Geometry: final body of the model. Coordinates: model frame, mm. A direction names the side the tool comes from. Give positions to 0.01 mm unless a question says otherwise; leave off trailing zeros. Order: outer loops, then holes, each group sorted by start corner. A loop starts at its lowest first (then second) coordinate and runs counter-clockwise, first axis right, second up. Notation, with made-up numbers: (83.25, 17) - (134.25, 17) arc R34 ccw to (134.25, 50) - close; hole circle Ø7 at (30.5, 56). An arc over 180 degrees is marked (long way). One line per item, written item: value.
```python
from build123d import *

# Parameters (mm, degrees)
F1_DEPTH = 12.7
F2_DEPTH = 25.4
F3_DEPTH = 50.8


with BuildPart() as f1:
    # F0 (on Front) → F1 (new body)
    with BuildSketch(Plane.XZ):
        Polygon((23.827744, -32.507298), (27.511551, -30.380452), (11.636551, -2.884145), (7.952744, -5.010992), (-7.922256, -32.507298), align=None)
        Polygon((27.511551, -30.380452), (32.624925, -29.077077), (18.205816, -4.102446), (11.636551, -2.884145), align=None)
    extrude(amount=-F1_DEPTH)

    # F0 (on Front) → F2 (join)
    with BuildSketch(Plane.XZ):
        with BuildLine():
            Line((32.624925, -29.077077), (36.2911, -22.727077))
            Line((36.2911, -22.727077), (23.705077, -0.927446))
            ThreePointArc((23.705077, -0.927446), (24.022261, -1.693196), (24.130446, -2.514946))
            ThreePointArc((24.130446, -2.514946), (21.777197, -5.581761), (18.205816, -4.102446))
            Line((18.205816, -4.102446), (32.624925, -29.077077))
        make_face()
    extrude(amount=-F2_DEPTH)

    # F0 (on Front) → F3 (join)
    with BuildSketch(Plane.XZ):
        with BuildLine():
            ThreePointArc((24.130446, -2.514946), (24.022261, -1.693196), (23.705077, -0.927446))
            ThreePointArc((23.705077, -0.927446), (19.367946, 0.234685), (18.205816, -4.102446))
            ThreePointArc((18.205816, -4.102446), (21.777197, -5.581761), (24.130446, -2.514946))
        make_face()
    extrude(amount=-F3_DEPTH)


solid = f1.part
```
1) Section D-D, the plane y = 23. Return loops of the section in (x, z) (3 decimals), then the cut area to 3 significant figures.
Answers below:
outline: (18.206, -4.102) - (32.625, -29.077) - (36.291, -22.727) - (23.705, -0.927) arc R3.175 ccw to start
area: 187 mm^2
2) Section C-C, the plane z = -25. Return loops of the section in (x, y), then the cut area to 3 significant figures.
Answers below:
outline: (-3.59, 0) - (34.98, 0) - (34.98, 25.4) - (30.27, 25.4) - (30.27, 12.7) - (-3.59, 12.7) - close
area: 550 mm^2
3) Section B-B, the plane x = 22. Return loops of the section in (y, z), then the cut area to 3 significant figures.
Answers below:
outline: (0, -32.51) - (12.7, -32.51) - (12.7, -10.67) - (25.4, -10.67) - (25.4, -5.51) - (50.8, -5.51) - (50.8, 0.48) - (0, 0.48) - close
area: 713 mm^2
4) First-contact query: pin 1 (1.5 mm diameter, centred on x = 2, z = -25.5, fed in from +Y); pin 2 (9 mm diameter, centred on x = 22, z = -18, fed in from +Y); pin 3 (1.5 mm diameter, centred on y = 40, z = -6.5, fed in from -X); pin 4 (10 mm diameter, centred on y = 19, z = -7.5, fed in from -X). Flat tips, straight axial feed; report the tip coordinate or a pass-through.
Answers below:
pin 1: y = 12.7
pin 2: y = 25.4
pin 3: through
pin 4: x = 17.78
5) Mould query, pull axis X, two halves, no side actions, for faces 1 (the face through (30.1, 12.5, -12)), 2 (the face through (12, 12.7, -21)), 3 (the face through (14.967, 6.261, -3.502)). Classes: released by +X, released by -X, zero draft, split by the parting line, or undercut.
Answers below:
face 1: released by +X
face 2: zero draft
face 3: undercut
6) Section A-A, the plane y = 12. Return loops of the section in (x, z) (3 decimals).
Answers below:
outline: (-7.922, -32.507) - (23.828, -32.507) - (27.512, -30.38) - (32.625, -29.077) - (36.291, -22.727) - (23.705, -0.927) arc R3.175 ccw to (18.206, -4.102) - (11.637, -2.884) - (7.953, -5.011) - close
7) Material intervals for line 1 along Y through (x, z) = (28, -26); line 2 along X through (y, z) = (33, -2.5); line 3 along Y through (x, z) = (28.5, -14.5), sorted ascending.
Answers below:
line 1: 0 to 12.7
line 2: 17.78 to 24.13
line 3: 0 to 25.4
8) Set-up query: faces 4 (the face through (34.43, 12.52, -25.95)), 5 (the face through (25.31, 18.96, -16.41)). Return all of +Z, -Z, +X, -X, +Y, -Y with unobstructed straight access to the full face (end or side cutting, diameter ignored); none if empty.
Answers below:
face 4: -Z, +X, +Y, -Y
face 5: -Z, -X, +Y
